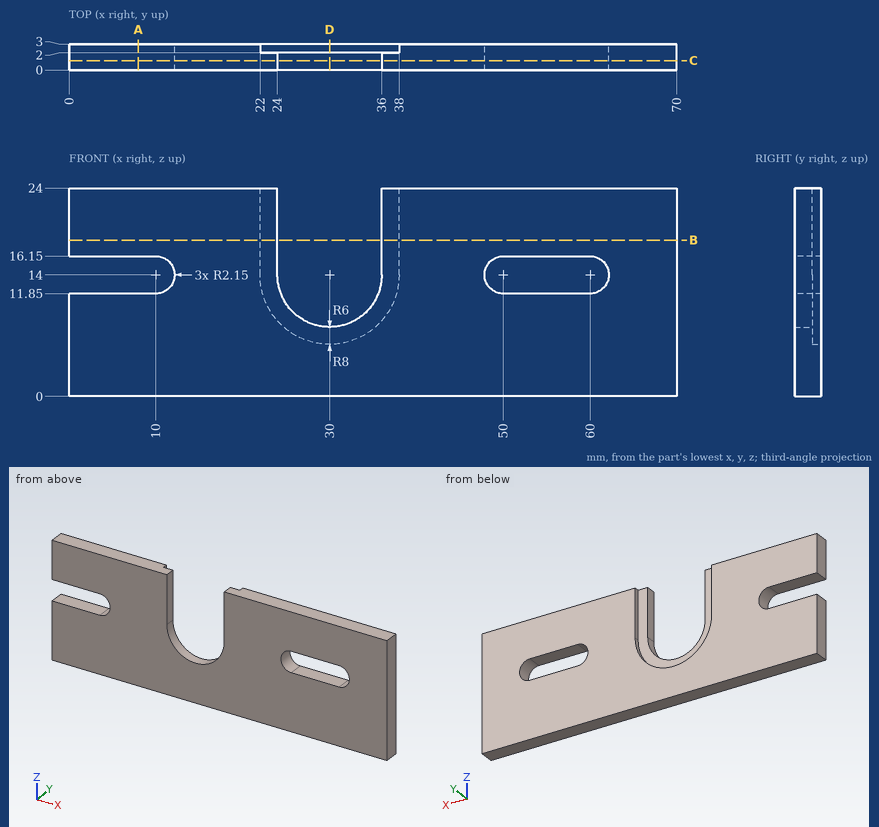
Geometry check sheet. Reference: drawing and pictorial views, mm from the part's lowest x, y, z. Give positions to 0.01 mm unless a question says otherwise; leave off trailing zeros. Order: outer loops, then holes, each group sorted by start corner. A loop starts at its lowest first (then second) coordinate and runs counter-clockwise, first axis right, second up. Notation, with made-up numbers: M 48.5,-5 L 74.5,-5 A14 cw 74.5,-1 Z; hole C 26.25,-37 d7. An arc over 180 degrees is marked long. Answer in a Markdown table with one row per item.
1) Cross-section at C-C, the plane y = 1.1. Enter the section's corners in (x, z).
Filled sheet:
| item | result |
|---|---|
| outline | M 0,0 L 70,0 L 70,24 L 36,24 L 36,14 A6 cw 24,14 L 24,24 L 0,24 L 0,16.15 L 10,16.15 A2.15 cw 10,11.85 L 0,11.85 Z; hole M 50,11.85 L 60,11.85 A2.15 ccw 60,16.15 L 50,16.15 A2.15 ccw Z |
2) Cross-section at B-B, the plane z = 18. Enter the section's corners in (x, y), plus the area to 3 significant figures.
Filled sheet:
| item | result |
|---|---|
| outline | M 0,0 L 24,0 L 24,2 L 22,2 L 22,3 L 0,3 Z; M 36,0 L 70,0 L 70,3 L 38,3 L 38,2 L 36,2 Z |
| area | 170 mm2 |
3) Thickness scan on L1, parallel to Z at x = 6, y = 2.45; L2, parallel to X at y = 2.1, z = 22.5; L3, parallel to X at y = 1.85, z = 16.75. Record the ranges inside material, lowest first. Write a range as [from, to].
Filled sheet:
| item | result |
|---|---|
| L1 | z = [0, 11.85], [16.15, 24] |
| L2 | x = [0, 22], [38, 70] |
| L3 | x = [0, 24], [36, 70] |
4) Cross-section at D-D, the plane x = 30. Enter the section's corners in (y, z), plus the area to 3 significant figures.
Filled sheet:
| item | result |
|---|---|
| outline | M 0,0 L 3,0 L 3,6 L 2,6 L 2,8 L 0,8 Z |
| area | 22.0 mm2 |
5) Cross-section at A-A, the plane x = 8. Enter the section's corners in (y, z).
Filled sheet:
| item | result |
|---|---|
| outline | M 0,0 L 3,0 L 3,11.85 L 0,11.85 Z; M 0,16.15 L 3,16.15 L 3,24 L 0,24 Z |
